Read the model definition and answer for the solid it produces. Units are mm, in the model's axes. A direction names the side the tool comes from. Coordinates: 2 decimals unless noted, no trailing zeros. Write each loop counter-clockwise with the first axis right and the second up, starting at its lowest first coordinate (ties: lowest second). Pieces come first, ordered by that corner, then holes.
(1) Section A-A on z = -4 is taken. Write down the section's boundary in (x, y), then the cut area to 3 significant figures.
(2) Which of the six approach directions +Z, -Z, +X, -X, +Y, -Y give full straight-line access (tool end or side, diameter ignored) to faces 4 (the conical face through (62.596, -1.261, 33.615)), 5 (the cylindrical face through (3.01, -0.01, 32.15)), 6 (the flat face through (60, 0, 0)), 7 (the flat face through (0, 0, -13))?
(3) Section B-B on y = 0 is taken. Write down the section's boundary in (x, z).
(4) Section C-C on x = 22.5 is taken. Write down the section's boundary in (y, z).
(5) The mould has two halves that part along Y. Classify faces 1 (the cylindrical face through (2.5, 0.1, -12.7)), 2 (the flat face through (63, 2.5, 3)), 3 (the flat face through (-1.3, 1, -0.2)): +Y half, -Y half, draft (parallel to the pull), parting line (faces both ways), or undercut.
(6) Find the intervals of material crossed by probe 1 along Y at (x, z) = (63, 24.5); probe 2 along X at (y, z) = (0.25, -8); probe 3 along Z at (x, y) = (28, -1.3), in increasing order.
(7) Given pin 1 (1 mm diameter, centred on x = 32.5, y = 0, fed in from -Z); pin 2 (1 mm diameter, centred on y = 0, z = 3, fed in from +X); pin 3 (2 mm diameter, centred on y = 0.5, z = 12.5, fed in from -X), each flat-ended and moving along its own axis, determine where each tip first touches the part or whether it passes through.
from build123d import *

# Parameters (mm, degrees)
ENL_V_MAT_EXTRU_1_DEPTH      = 79.42671739
ENL_V_MAT_EXTRU_1_DEPTH_BACK = 79.42671739


with BuildPart() as part:
    # Balayage1: sweep along a path in Esquisse2
    with BuildLine(Plane(origin=(0, 0, 0), x_dir=(1, 0, 0), z_dir=(0, 1, 0))) as balayage1_path:
        Line((0, 0), (0, 25))
        ThreePointArc((0, 25), (2.928932188, 32.071067812), (10, 35))
        Line((10, 35), (50, 35))
        ThreePointArc((50, 35), (57.071067812, 32.071067812), (60, 25))
        Line((60, 25), (60, -25))
        ThreePointArc((60, -25), (57.071067812, -32.071067812), (50, -35))
        Line((50, -35), (10, -35))
        ThreePointArc((10, -35), (2.928932188, -32.071067812), (0, -25))
        Line((0, -25), (0, -0.5))
    # Esquisse1 → Balayage1 (sweep)
    with BuildSketch(Plane.XY):
        with BuildLine():
            Line((0, -1), (0, 1))
            Line((0, 1), (-5, 1))
            Line((-5, 1), (-6.5, 2.5))
            Line((-6.5, 2.5), (0, 2.5))
            ThreePointArc((0, 2.5), (2.5, 0), (0, -2.5))
            Line((0, -2.5), (-6.5, -2.5))
            Line((-6.5, -2.5), (-5, -1))
            Line((-5, -1), (0, -1))
        make_face()
    sweep(path=balayage1_path.line)

    # Esquisse3 → Enlèv. mat.-Extru.1 (cut, two sides: drawn at the far end of the back side and taken through both)
    with BuildSketch(Plane(origin=(0, 0, 0), x_dir=(0, 0, -1), z_dir=(1, 0, 0)).offset(-ENL_V_MAT_EXTRU_1_DEPTH_BACK)):
        Polygon((-40, -1), (-43.95658592, -1), (-43.95658592, -4.130810218), (-39.042815259, -4.130810218), align=None)
    extrude(amount=ENL_V_MAT_EXTRU_1_DEPTH + ENL_V_MAT_EXTRU_1_DEPTH_BACK, mode=Mode.SUBTRACT)


solid = part.part
Response:
1. outline: (-6.5, -2.5) - (0, -2.5) arc R2.5 ccw to (0, 2.5) - (-6.5, 2.5) - (-5, 1) - (0, 1) - (0, -1) - (-5, -1) - close; (60, -2.5) - (66.5, -2.5) - (65, -1) - (60, -1) - (60, 1) - (65, 1) - (66.5, 2.5) - (60, 2.5) arc R2.5 ccw to start
1. area: 54.1 mm2
2. face 4: +Z, +X
2. face 5: +Z, -X
2. face 6: +Z, -Z, +X
2. face 7: +Z, -Z, -X
3. outline: (0, -25) arc R10 ccw to (10, -35) - (50, -35) arc R10 ccw to (60, -25) - (60, 25) arc R10 ccw to (50, 35) - (10, 35) arc R10 ccw to (0, 25) - (0, 0.5) - (2.5, 0.5) - (2.5, 25) arc R7.5 cw to (10, 32.5) - (50, 32.5) arc R7.5 cw to (57.5, 25) - (57.5, -25) arc R7.5 cw to (50, -32.5) - (10, -32.5) arc R7.5 cw to (2.5, -25) - (2.5, 0) - (0, 0) - close
4. outline: (-2.5, -41.5) - (-1, -40) - (-1, -35) - (1, -35) - (1, -40) - (2.5, -41.5) - (2.5, -35) arc R2.5 ccw to (-2.5, -35) - close; (-2.5, 35) arc R2.5 ccw to (2.5, 35) - (2.5, 41.5) - (1, 40) - (1, 35) - (-1, 35) - (-1, 40) - (-2.5, 39.54) - close
5. face 1: parting line
5. face 2: +Y half
5. face 3: undercut
6. probe 1: y = -2.5 to -1, 1 to 2.5
6. probe 2: x = 0 to 2.49, 57.51 to 60
6. probe 3: z = -40.3 to -32.86, 32.86 to 39.91
7. pin 1: stops at z = -35
7. pin 2: stops at x = 60
7. pin 3: stops at x = -5.5
